Check sheet for the modelled part. Datum: model origin and axes. Units: mm. Face numbers are marked on the shaded views. A direction names the side the tool comes from. Coordinates: 2 decimals unless noted, no trailing zeros. Write each loop counter-clockwise with the first axis right and the second up, starting at its lowest first coordinate (ties: lowest second). Pieces come first, ordered by that corner, then holes. Notation, with made-up numbers: (-1, 34.25) -> (25, 34.25) arc R14 ccw to (25, 53.25) -> close; hole circle Ø9 at (0.5, -13). An arc over 180 degrees is marked (long way). Put each result on its own line as item: value.
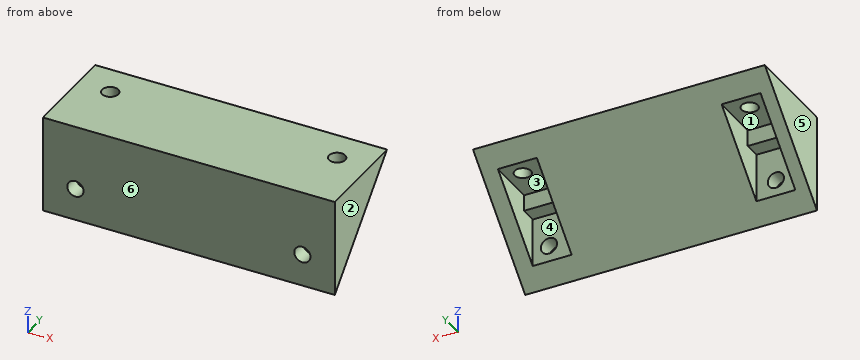
```python
from build123d import *

# Parameters (mm, degrees)
BOSS_EXTRUDE1_DEPTH = 45
CUT_EXTRUDE1_START  = -5
SKETCH2_W           = 12
SKETCH2_H           = 20
CUT_EXTRUDE1_DEPTH  = 57.846584384
SKETCH3_R           = 2.5
CUT_EXTRUDE2_DEPTH  = 62.846584384


with BuildPart() as part:
    # Sketch1 → Boss-Extrude1 (new, symmetric)
    with BuildSketch(Plane(origin=(0, 0, 0), x_dir=(0, 0, -1), z_dir=(1, 0, 0))):
        Polygon((0, 0), (0, 30), (30, 0), align=None)
    extrude(amount=BOSS_EXTRUDE1_DEPTH, both=True)

    # Sketch2 → Cut-Extrude1 (cut, through all)
    with BuildSketch(Plane.XY.offset(CUT_EXTRUDE1_START)):
        with Locations((-35, 20)):
            Rectangle(SKETCH2_W, SKETCH2_H)
        with Locations((34, 20)):
            Rectangle(SKETCH2_W, SKETCH2_H)
    cut_extrude1 = extrude(amount=-CUT_EXTRUDE1_DEPTH, mode=Mode.SUBTRACT)

    # Sketch3 → Cut-Extrude2 (cut, through all)
    with BuildSketch(Plane.XY):
        with Locations((-35, 20)):
            Circle(SKETCH3_R)
        with Locations((35, 20)):
            Circle(SKETCH3_R)
    cut_extrude2 = extrude(amount=-CUT_EXTRUDE2_DEPTH, mode=Mode.SUBTRACT)

    # Mirror1: Cut-Extrude1, Cut-Extrude2 across plane
    add(cut_extrude1.mirror(Plane(origin=(0, 0, 0), x_dir=(0, -0.7071067811865477, 0.7071067811865474), z_dir=(0, -0.7071067811865476, -0.7071067811865476))), mode=Mode.SUBTRACT)
    add(cut_extrude2.mirror(Plane(origin=(0, 0, 0), x_dir=(0, -0.7071067811865477, 0.7071067811865474), z_dir=(0, -0.7071067811865476, -0.7071067811865476))), mode=Mode.SUBTRACT)


solid = part.part
```
Q1. Cross-section at A-A (z = -20). Record the cut outline in (x, y).
Recorded:
outline: (-45, 0) -> (-37.5, 0) -> (-37.5, 5) -> (-41, 5) -> (-41, 10) -> (-45, 10) -> close; (-32.5, 0) -> (32.5, 0) -> (32.5, 5) -> (28, 5) -> (28, 10) -> (-29, 10) -> (-29, 5) -> (-32.5, 5) -> close; (37.5, 0) -> (45, 0) -> (45, 10) -> (40, 10) -> (40, 5) -> (37.5, 5) -> close
Q2. Cross-section at D-D (y = 3.5). Record the cut outline in (x, z).
Recorded:
outline: (-45, -26.5) -> (45, -26.5) -> (45, 0) -> (-45, 0) -> close; hole circle Ø5 at (-35, -20); hole circle Ø5 at (35, -20)
Q3. Tool access check on the marked faces 1 and 2. Record the directions out of +Z, -Z, +X, -X, +Y, -Y that give a thin tool (end or side, any length) a straight path to the whole face; none if there is none.
Recorded:
face 1: -Z, +Y
face 2: +Z, -Z, +X, +Y, -Y
Q4. Cross-section at C-C (x = -35). Record the cut outline in (y, z), plus the area to 3 significant figures.
Recorded:
outline: (0, -30) -> (5, -25) -> (5, -22.5) -> (0, -22.5) -> close; (0, -17.5) -> (5, -17.5) -> (5, -10) -> (10, -10) -> (10, -5) -> (17.5, -5) -> (17.5, 0) -> (0, 0) -> close; (22.5, -5) -> (25, -5) -> (30, 0) -> (22.5, 0) -> close
area: 225 mm2
Q5. Cross-section at B-B (y = 20). Record the cut outline in (x, z), plus the area to 3 significant figures.
Recorded:
outline: (-45, -10) -> (-41, -10) -> (-41, -5) -> (-37.5, -5) -> (-37.5, 0) -> (-45, 0) -> close; (-32.5, -5) -> (-29, -5) -> (-29, -10) -> (28, -10) -> (28, -5) -> (32.5, -5) -> (32.5, 0) -> (-32.5, 0) -> close; (37.5, -5) -> (40, -5) -> (40, -10) -> (45, -10) -> (45, 0) -> (37.5, 0) -> close
area: 730 mm2
Q6. Depth check by flat-ended pin: P1, Ø6, axis at x = 32, y = 17.5, coming from the -Z side; P2, Ø1, axis at x = 22, z = -21, coming from the +Y side; P3, Ø5.5, axis at x = -32.5, z = -8.5, coming from the +Y side. Enter the tip coordinate at first touch or a pass-through.
Recorded:
P1: stops at z = -5
P2: stops at y = 9.5
P3: stops at y = 10
Q7. Mould release check, pull along X, two halves, no side actions. Record for the marked faces 3, 4, 5 and 6: released by +X, released by -X, zero draft, split by the parting line, or undercut.
Recorded:
face 3: undercut
face 4: undercut
face 5: released by -X
face 6: zero draft
Q8. Material ranges on line 1 along X through (y, z) = (2, -20); line 2 along X through (y, z) = (16.5, -11.5); line 3 along Z through (x, y) = (-35, 3.2), recorded low to high.
Recorded:
line 1: x = -45 to -37.5, -32.5 to 32.5, 37.5 to 45
line 2: x = -45 to -41, -29 to 28, 40 to 45
line 3: z = -26.8 to -22.5, -17.5 to 0
